The listing builds one solid part. Answer for the finished solid, in the listing's coordinates (mm). Give positions to 0.01 mm unless a question says otherwise; leave off trailing zeros. Order: outer loops, then holes, each group sorted by start corner. A loop starts at its lowest first (then second) coordinate and runs counter-clockwise, first axis right, second up. Notation, with made-up numbers: (-1.75, -26.75) - (22.25, -26.75) arc R11 cw to (22.25, -20.75) - close; hole circle Ø5 at (47, 36). An arc over 180 degrees is marked (long way). Answer as CSV lines item,"result". Start each with the question number.
1. Section A-A on z = 0.75 is taken. Give the vertices of the cut face in (x, y) (3 decimals).
2. Section B-B on y = 82 is taken. Give the vertices of the cut face in (x, z) (3 decimals), and give its area (3 significant figures).
3. Consider line 1 along Y through (x, z) = (0, 8.4); line 2 along Z through (x, y) = (1.5, 117.5) (3 decimals); line 3 along X through (y, z) = (302, 4.5) (3 decimals). Determine where each line is inside the solid, lowest interval first. Write a range as [from, to].
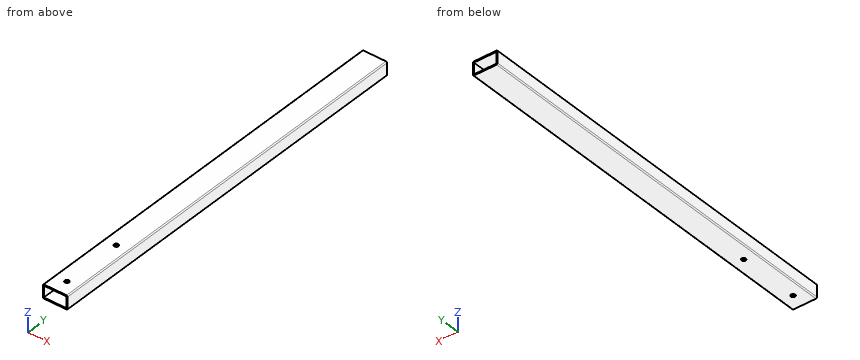
from build123d import *

# Parameters (mm, degrees)
SKETCH1_W               = 34.29
SKETCH1_H               = 19.05
SKETCH1_W_2             = 31.75
SKETCH1_H_2             = 15.748
BOSS_EXTRUDE1_DEPTH     = 550
FILLET1_R               = 1.5
CUT_EXTRUDE1_DEPTH      = 551.59681576
CUT_EXTRUDE1_DEPTH_BACK = 551.59681576
SKETCH2_R               = 3


with BuildPart() as part:
    # Sketch1 → Boss-Extrude1 (new body)
    with BuildSketch(Plane(origin=(0, 0, 0), x_dir=(1, 0, 0), z_dir=(0, 1, 0))):
        Rectangle(SKETCH1_W, SKETCH1_H)
        Rectangle(SKETCH1_W_2, SKETCH1_H_2, mode=Mode.SUBTRACT)
    extrude(amount=BOSS_EXTRUDE1_DEPTH)

    # Fillet1
    fillet1_edges = [part.edges().sort_by_distance(p)[0] for p in [
        (17.145, 275, 9.525),
        (-17.145, 275, 9.525),
        (-17.145, 275, -9.525),
        (17.145, 275, -9.525),
    ]]
    fillet(fillet1_edges, radius=FILLET1_R)

    # Sketch2 → Cut-Extrude1 (cut, two sides: drawn at the far end of the back side and taken through both)
    with BuildSketch(Plane.XY.offset(9.525).offset(-CUT_EXTRUDE1_DEPTH_BACK)):
        with Locations(Location((0, 105, 0), (0, 0, 180))):
            Circle(SKETCH2_R)
        with Locations(Location((0, 20, 0), (0, 0, 180))):
            Circle(SKETCH2_R)
    extrude(amount=CUT_EXTRUDE1_DEPTH + CUT_EXTRUDE1_DEPTH_BACK, mode=Mode.SUBTRACT)


solid = part.part
Checks:
1,outline,"(-17.145, 0) - (-15.875, 0) - (-15.875, 550) - (-17.145, 550) - close; (15.875, 0) - (17.145, 0) - (17.145, 550) - (15.875, 550) - close"
2,outline,"(-17.145, -8.025) arc R1.5 ccw to (-15.645, -9.525) - (15.645, -9.525) arc R1.5 ccw to (17.145, -8.025) - (17.145, 8.025) arc R1.5 ccw to (15.645, 9.525) - (-15.645, 9.525) arc R1.5 ccw to (-17.145, 8.025) - close; hole (-15.875, -7.874) - (15.875, -7.874) - (15.875, 7.874) - (-15.875, 7.874) - close"
2,area,"151 mm²"
3,line 1,"y = [0, 17], [23, 102], [108, 550]"
3,line 2,"z = [-9.525, -7.874], [7.874, 9.525]"
3,line 3,"x = [-17.145, -15.875], [15.875, 17.145]"
